Input: part model. Units: mm. Frame: model coordinates. Face numbers are marked on the shaded views. Round coordinates to 2 decimals unless told otherwise and drop trailing zeros. Order: outer loops, then holes, each group sorted by start corner. A loop starts at its lowest first (then second) coordinate and runs counter-clockwise, first axis right, second up.
Item 1: Cut plane B-B on y = 16. Output: boundary loops of the cut face in (x, z).
Item 2: Mould query, pull axis X, two halves, no side actions, for the marked faces 1 and 2. Classes: released by +X, released by -X, zero draft, split by the parting line, or undercut.
Item 3: Line query: L1, parallel to X at y = -8, z = 6; L2, parallel to Y at x = 12.5, z = 21; L3, parallel to X at y = 21, z = 23.25. Output: solid intervals per line, ascending.
Item 4: Cut plane A-A on z = 9.25. Output: boundary loops of the cut face in (x, y).
Item 5: Cut plane C-C on x = 7.5. Give the number of separate pieces and of enclosed holes in the cut face, then the cut area to 3 significant figures.
Item 6: First-contact query: pin 1 (3 mm diameter, centred on x = 14, z = 4, fed in from -Y); pin 2 (3 mm diameter, centred on y = -4, z = 12.5, fed in from +X); pin 3 (10 mm diameter, centred on x = -9, z = 20.5, fed in from +Y). Flat tips, straight axial feed; report the tip coordinate or a pass-through.
```python
from build123d import *

# Parameters (mm, degrees)
F0_R     = 37.5
F1_DEPTH = 3
F2_DEPTH = 25


with BuildPart() as f1:
    # F0 (on Top) → F1 (new body)
    with BuildSketch(Plane.XY):
        with BuildLine():
            ThreePointArc((11, -24), (7.778175, -16.221825), (0, -13))
            ThreePointArc((0, -13), (-7.778175, -31.778175), (11, -24))
        make_face()
        with BuildLine():
            ThreePointArc((11, 24), (-7.778175, 31.778175), (0, 13))
            ThreePointArc((0, 13), (7.778175, 16.221825), (11, 24))
        make_face()
        Circle(F0_R)
        with BuildLine():
            ThreePointArc((11, -24), (-7.778175, -31.778175), (0, -13))
            ThreePointArc((0, -13), (7.778175, -16.221825), (11, -24))
        make_face(mode=Mode.SUBTRACT)
        with BuildLine():
            ThreePointArc((-4.511195, 36.723958), (-13.469182, 24.911673), (-6.184658, 12))
            ThreePointArc((-6.184658, 12), (-13.5, 0), (-6.184658, -12))
            ThreePointArc((-6.184658, -12), (-13.469182, -24.911673), (-4.511195, -36.723958))
            ThreePointArc((-4.511195, -36.723958), (-37, 0), (-4.511195, 36.723958))
        make_face(mode=Mode.SUBTRACT)
        with BuildLine():
            ThreePointArc((0, 11), (7.778175, 7.778175), (11, 0))
            ThreePointArc((11, 0), (7.778175, -7.778175), (0, -11))
            ThreePointArc((0, -11), (-11, 0), (0, 11))
        make_face(mode=Mode.SUBTRACT)
        with BuildLine():
            ThreePointArc((6.184658, -12), (13.5, 0), (6.184658, 12))
            ThreePointArc((6.184658, 12), (13.469182, 24.911673), (4.511195, 36.723958))
            ThreePointArc((4.511195, 36.723958), (37, 0), (4.511195, -36.723958))
            ThreePointArc((4.511195, -36.723958), (13.469182, -24.911673), (6.184658, -12))
        make_face(mode=Mode.SUBTRACT)
        with BuildLine():
            ThreePointArc((11, 24), (7.778175, 16.221825), (0, 13))
            ThreePointArc((0, 13), (-7.778175, 31.778175), (11, 24))
        make_face(mode=Mode.SUBTRACT)
    extrude(amount=F1_DEPTH)

    # F0 (on Top) → F2 (join)
    with BuildSketch(Plane.XY):
        with BuildLine():
            ThreePointArc((11, -24), (7.778175, -16.221825), (0, -13))
            ThreePointArc((0, -13), (-7.778175, -31.778175), (11, -24))
        make_face()
        with BuildLine():
            ThreePointArc((11, 24), (-7.778175, 31.778175), (0, 13))
            ThreePointArc((0, 13), (7.778175, 16.221825), (11, 24))
        make_face()
        Circle(F0_R)
        with BuildLine():
            ThreePointArc((11, -24), (-7.778175, -31.778175), (0, -13))
            ThreePointArc((0, -13), (7.778175, -16.221825), (11, -24))
        make_face(mode=Mode.SUBTRACT)
        with BuildLine():
            ThreePointArc((-4.511195, 36.723958), (-13.469182, 24.911673), (-6.184658, 12))
            ThreePointArc((-6.184658, 12), (-13.5, 0), (-6.184658, -12))
            ThreePointArc((-6.184658, -12), (-13.469182, -24.911673), (-4.511195, -36.723958))
            ThreePointArc((-4.511195, -36.723958), (-37, 0), (-4.511195, 36.723958))
        make_face(mode=Mode.SUBTRACT)
        with BuildLine():
            ThreePointArc((0, 11), (7.778175, 7.778175), (11, 0))
            ThreePointArc((11, 0), (7.778175, -7.778175), (0, -11))
            ThreePointArc((0, -11), (-11, 0), (0, 11))
        make_face(mode=Mode.SUBTRACT)
        with BuildLine():
            ThreePointArc((6.184658, -12), (13.5, 0), (6.184658, 12))
            ThreePointArc((6.184658, 12), (13.469182, 24.911673), (4.511195, 36.723958))
            ThreePointArc((4.511195, 36.723958), (37, 0), (4.511195, -36.723958))
            ThreePointArc((4.511195, -36.723958), (13.469182, -24.911673), (6.184658, -12))
        make_face(mode=Mode.SUBTRACT)
        with BuildLine():
            ThreePointArc((11, 24), (7.778175, 16.221825), (0, 13))
            ThreePointArc((0, 13), (-7.778175, 31.778175), (11, 24))
        make_face(mode=Mode.SUBTRACT)
    extrude(amount=F2_DEPTH)


solid = f1.part
```
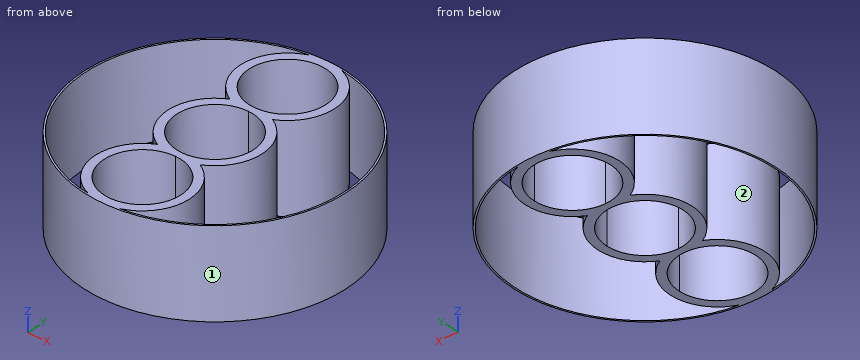
From the geometry:
1. outline: (-33.92, 0) - (-33.36, 0) - (-33.36, 25) - (-33.92, 25) - close; (-10.87, 0) - (-7.55, 0) - (-7.55, 25) - (-10.87, 25) - close; (7.55, 0) - (10.87, 0) - (10.87, 25) - (7.55, 25) - close; (33.36, 0) - (33.92, 0) - (33.92, 25) - (33.36, 25) - close
2. face 1: split by the parting line
2. face 2: undercut
3. L1: x = -36.64 to -36.12, -10.87 to -7.55, 7.55 to 10.87, 36.12 to 36.64
3. L2: y = -35.36 to -34.82, -29.1 to -18.9, -5.1 to 5.1, 18.9 to 29.1, 34.82 to 35.36
3. L3: x = -31.07 to -30.46, -13.16 to -10.58, 10.58 to 13.16, 30.46 to 31.07
4. outline: circle Ø75 at (0, 0); hole (-6.18, -12) arc R13.5 cw to (-6.18, 12) arc R13.5 cw to (-4.51, 36.72) arc R37 ccw to (-4.51, -36.72) arc R13.5 cw to start; hole (0, -13) arc R11 ccw (long way) to (11, -24) arc R11 ccw to start; hole (0, -11) arc R11 ccw to (11, 0) arc R11 ccw to (0, 11) arc R11 ccw to start; hole (0, 13) arc R11 ccw to (11, 24) arc R11 ccw (long way) to start; hole (4.51, -36.72) arc R37 ccw to (4.51, 36.72) arc R13.5 cw to (6.18, 12) arc R13.5 cw to (6.18, -12) arc R13.5 cw to start
5. separate pieces: 8
5. enclosed holes: 0
5. area: 502 mm2
6. pin 1: stops at y = -35.36
6. pin 2: stops at x = 37.42
6. pin 3: stops at y = 37.29
